Geometry: see drawing. Coordinates: mm, zero at the bounding-box minimum. A direction names the side the tool comes from. Give positions to 0.01 mm unless a question says otherwise; leave off trailing zeros. Loops run counter-clockwise (first coordinate to the right, second up) from the corner with the lowest first, then second, coordinate; pieces in that order, holes last. Notation, with made-up numbers: (-35.5, 14.5) -> (16.5, 14.5) arc R31 cw to (16.5, 46.5) -> close; hole circle Ø11 at (-8.5, -20). An arc over 180 degrees is marked (long way). Return JSON: item names as keys, results as strings. Group by question number.
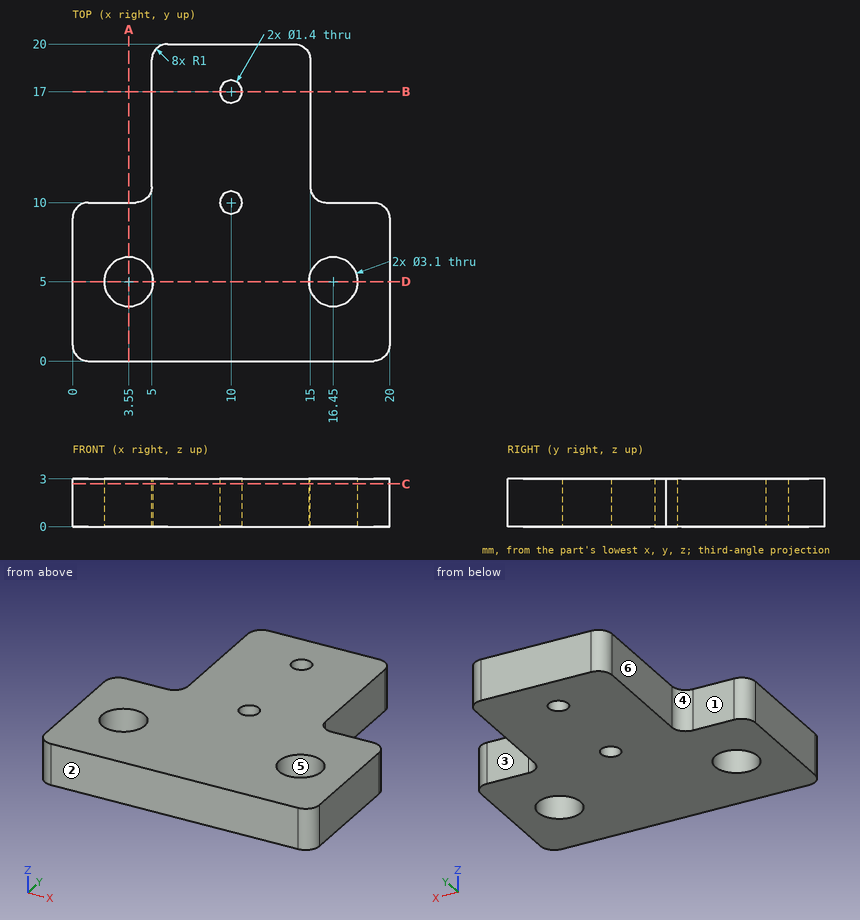
1) Contact query for flat-ended pins moving along their axis: P1, Ø0.8, axis at x = 10, y = 17, coming from the +Z side; P2, Ø0.9, axis at y = 14.5, z = 2, coming from the +X side; P3, Ø1.5, axis at x = 3, z = 2, coming from the +Y side; P4, Ø5, axis at x = 7, y = 4, coming from the -Z side. Output: stop coordinate, or through.
2) Cut plane A-A on x = 3.55. Return loops of the section in (y, z).
3) Material intervals for line 1 (Y direction, x = 10, z = 2); line 2 (Y direction, x = 16.45, z = 1); line 3 (X direction, y = 17, z = 1.55), sorted ascending.
4) Mould query, pull axis Y, two halves, no side actions, for the marked faces 4, 5 and 6. Classes: released by +Y, released by -Y, zero draft, split by the parting line, or undercut.
5) Reachability of the marked faces 1, 2 and 3 from +Z, -Z, +X, -X, +Y, -Y: full face, straight path, thin tool, end or side. Return the list, or none.
6) Cut plane C-C on z = 2.7. Return loops of the section in (x, y).
7) Cut plane D-D on y = 5. Return loops of the section in (x, z).
8) Cut plane B-B on y = 17. Return loops of the section in (x, z), then the cut area to 3 significant figures.
Calculated:
{
 "1": {"P1": "through", "P2": "x = 15", "P3": "y = 10", "P4": "z = 0"},
 "2": {"outline": "(0, 0) -> (3.45, 0) -> (3.45, 3) -> (0, 3) -> close; (6.55, 0) -> (10, 0) -> (10, 3) -> (6.55, 3) -> close"},
 "3": {"line 1": "0 to 9.3, 10.7 to 16.3, 17.7 to 20", "line 2": "0 to 3.45, 6.55 to 10", "line 3": "5 to 9.3, 10.7 to 15"},
 "4": {"face 4": "released by +Y", "face 5": "undercut", "face 6": "zero draft"},
 "5": {"face 1": "+Z, -Z, -X, +Y", "face 2": "+Z, -Z, +X, -X, -Y", "face 3": "+Z, -Z, +X, +Y"},
 "6": {"outline": "(0, 1) arc R1 ccw to (1, 0) -> (19, 0) arc R1 ccw to (20, 1) -> (20, 9) arc R1 ccw to (19, 10) -> (16, 10) arc R1 cw to (15, 11) -> (15, 19) arc R1 ccw to (14, 20) -> (6, 20) arc R1 ccw to (5, 19) -> (5, 11) arc R1 cw to (4, 10) -> (1, 10) arc R1 ccw to (0, 9) -> close; hole circle Ø3.1 at (3.55, 5); hole circle Ø1.4 at (10, 10); hole circle Ø1.4 at (10, 17); hole circle Ø3.1 at (16.45, 5)"},
 "7": {"outline": "(0, 0) -> (2, 0) -> (2, 3) -> (0, 3) -> close; (5.1, 0) -> (14.9, 0) -> (14.9, 3) -> (5.1, 3) -> close; (18, 0) -> (20, 0) -> (20, 3) -> (18, 3) -> close"},
 "8": {"outline": "(5, 0) -> (9.3, 0) -> (9.3, 3) -> (5, 3) -> close; (10.7, 0) -> (15, 0) -> (15, 3) -> (10.7, 3) -> close", "area": "25.8 mm2"}
}
